Design review of the part built by this model. Coordinates are the model's own, in mm. Coordinates: 2 decimals unless noted, no trailing zeros. Order: outer loops, then holes, each group sorted by start corner. A loop starts at its lowest first (then second) coordinate and runs counter-clockwise, first axis right, second up. Notation, with made-up numbers: (68.25, -0.75) -> (109.25, -0.75) arc R17 cw to (109.25, 32.25) -> close; hole circle Ø3 at (-2, -26.5). An arc over 180 degrees is marked (long way). Use a Markdown table: item, result. Add a question column.
Q1. Add section A-A (x = -32). State the section outline as (y, z) points.
Q2. Add section B-B (z = 5.5). State the section outline as (x, y) points.
Q3. Add section C-C (y = 0.7). State the section outline as (x, z) points, then the cut area to 3 significant figures.
Q4. Wall thickness on probe 1 along Z at (x, y) = (-26, 0.85); probe 2 along X at (y, z) = (1.9, -5.5); probe 3 along Z at (x, y) = (-32, 1.05): over which ranges is each line inside the solid? List them lowest first.
from build123d import *

# Parameters (mm, degrees)
SKETCH1_W           = 72
SKETCH1_H           = 38.5
SKETCH1_R           = 1.5
SKETCH1_W_2         = 54
SKETCH1_H_2         = 27
BOSS_EXTRUDE1_DEPTH = 3
FILLET1_R           = 3


with BuildPart() as part:
    # Sketch1 → Boss-Extrude1 (new body)
    with BuildSketch(Plane(origin=(0, 0, 0), x_dir=(1, 0, 0), z_dir=(0, 1, 0))):
        Rectangle(SKETCH1_W, SKETCH1_H)
        with Locations((-32, 0)):
            Circle(SKETCH1_R, mode=Mode.SUBTRACT)
        with Locations((32, 0)):
            Circle(SKETCH1_R, mode=Mode.SUBTRACT)
        Rectangle(SKETCH1_W_2, SKETCH1_H_2, mode=Mode.SUBTRACT)
    extrude(amount=BOSS_EXTRUDE1_DEPTH)

    # Fillet1
    fillet1_edges = [part.edges().sort_by_distance(p)[0] for p in [
        (-36, 1.5, -19.25),
        (36, 1.5, -19.25),
        (36, 1.5, 19.25),
        (-36, 1.5, 19.25),
    ]]
    fillet(fillet1_edges, radius=FILLET1_R)


solid = part.part
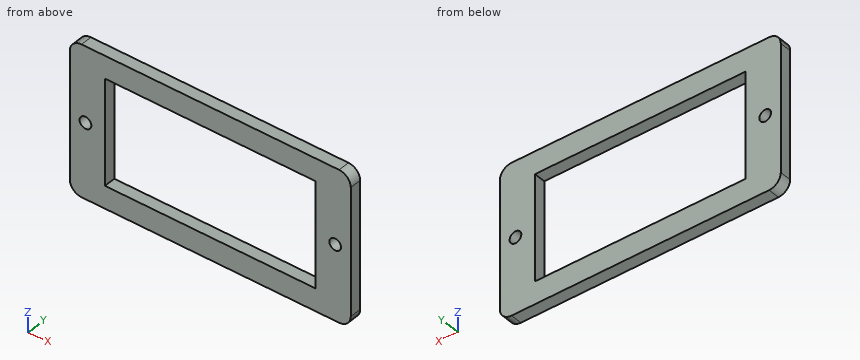
Established:
| question | item | result |
|---|---|---|
| 1 | outline | (0, -19.25) -> (3, -19.25) -> (3, -1.5) -> (0, -1.5) -> close; (0, 1.5) -> (3, 1.5) -> (3, 19.25) -> (0, 19.25) -> close |
| 2 | outline | (-36, 0) -> (-27, 0) -> (-27, 3) -> (-36, 3) -> close; (27, 0) -> (36, 0) -> (36, 3) -> (27, 3) -> close |
| 3 | outline | (-36, -16.25) arc R3 ccw to (-33, -19.25) -> (33, -19.25) arc R3 ccw to (36, -16.25) -> (36, 16.25) arc R3 ccw to (33, 19.25) -> (-33, 19.25) arc R3 ccw to (-36, 16.25) -> close; hole circle Ø3 at (-32, 0); hole (-27, -13.5) -> (27, -13.5) -> (27, 13.5) -> (-27, 13.5) -> close; hole circle Ø3 at (32, 0) |
| 3 | area | 1,290 mm^2 |
| 4 | probe 1 | -19.25 to -13.5, 13.5 to 19.25 |
| 4 | probe 2 | -36 to -27, 27 to 36 |
| 4 | probe 3 | -19.25 to -1.5, 1.5 to 19.25 |
